Build history of the part. All positions in model axes, mm. Give positions to 0.01 mm unless a question says otherwise; leave off trailing zeros. Loops run counter-clockwise (first coordinate to the right, second up) from the corner with the lowest first, then second, coordinate; pieces in that order, holes last. Notation, with made-up numbers: (41.25, 37) - (54.25, 37) arc R16 cw to (54.25, 67) - close; hole circle Ø3 at (61, 35.25). An arc over 180 degrees is marked (long way). Return JSON: item names as keys, results as strings. Group by question number.
1) Mould opens along Y. For faces 1 (the face through (4.78, 21.526, 4.507)), 2 (the face through (16, 16, 5)), 3 (the face through (-24.18, -7.61, 1.68)) say: released by +Y, released by -Y, zero draft, split by the parting line, or undercut.
2) Drop flat-ended pins along their axis: pin 1 (1.5 mm diameter, centred on y = -8, z = 3, fed in from +X); pin 2 (1 mm diameter, centred on y = -8.5, z = 1.5, fed in from +X); pin 3 (1.5 mm diameter, centred on x = -4.5, z = 1.5, fed in from +Y). Give the stop position or say it passes through.
3) Slice it at A-A (x = 0). List the corners of the cut face in (y, z).
4) Drill centre lines: probe 1 along X at (y, z) = (0, 1.05); probe 2 along Y at (x, z) = (2.5, 4.5); probe 3 along Y at (x, z) = (0, 4.65). Where is each one in solid material? Low to high. Write a range as from..to.
```python
from build123d import *


with BuildPart() as f2:
    # F1 (on Front) → F2 (revolve)
    with BuildSketch(Plane.XZ):
        with BuildLine():
            Line((-25.35, 3.4), (-25.35, 0))
            Line((-25.35, 0), (-24.35, 1))
            Line((-24.35, 1), (-24.35, 3.403729))
            ThreePointArc((-24.35, 3.403729), (-24.172952, 3.825589), (-23.75, 4.000012))
            Line((-23.75, 4.000012), (-22.05, 4.000012))
            Line((-22.05, 4.000012), (-22.05, 5))
            Line((-22.05, 5), (-23.75, 5))
            ThreePointArc((-23.75, 5), (-24.881371, 4.531371), (-25.35, 3.4))
        make_face()
    revolve(axis=Axis((0, 0, 18.396249), (0, 0, 1)))


solid = f2.part
```
Results:
{
 "1": {"face 1": "undercut", "face 2": "zero draft", "face 3": "split by the parting line"},
 "2": {"pin 1": "x = 24.29", "pin 2": "x = 24.05", "pin 3": "y = 25.07"},
 "3": {"outline": "(-25.35, 0) - (-24.35, 1) - (-24.35, 3.4) arc R0.6 cw to (-23.75, 4) - (-22.05, 4) - (-22.05, 5) - (-23.75, 5) arc R1.6 ccw to (-25.35, 3.4) - close; (22.05, 4) - (23.75, 4) arc R0.6 cw to (24.35, 3.4) - (24.35, 1) - (25.35, 0) - (25.35, 3.4) arc R1.6 ccw to (23.75, 5) - (22.05, 5) - close"},
 "4": {"probe 1": "-25.35..-24.35, 24.35..25.35", "probe 2": "-24.79..-21.91, 21.91..24.79", "probe 3": "-24.75..-22.05, 22.05..24.75"}
}
